from build123d import *

# Parameters (mm, degrees)
F1_DEPTH = 48
F0_W     = 15
F0_H     = 30
F2_DEPTH = 10
F3_R     = 6


with BuildPart() as f1:
    # F0 (on Top) → F1 (new body)
    with BuildSketch(Plane.XY):
        Polygon((21, 30), (21, 10), (-21, 10), (-21, 30), (-31, 30), (-31, 0), (31, 0), (31, 30), align=None)
    extrude(amount=F1_DEPTH)

    # F0 (on Top) → F2 (join)
    with BuildSketch(Plane.XY):
        Polygon((46, 0), (31, 0), (-31, 0), (-46, 0), (-46, -18), (46, -18), align=None)
        with Locations((38.5, 15)):
            Rectangle(F0_W, F0_H)
        with Locations((-38.5, 15)):
            Rectangle(F0_W, F0_H)
    extrude(amount=F2_DEPTH)

    # F3
    f3_edges = [f1.edges().sort_by_distance(p)[0] for p in [
        (46, -18, 5),
        (-46, -18, 5),
    ]]
    fillet(f3_edges, radius=F3_R)


solid = f1.part
Source: CAD feature listing. Evaluate the final solid. Frame: model axes, mm. A direction names the side the tool comes from. Coordinates: 2 decimals unless noted, no trailing zeros. Loops run counter-clockwise (first coordinate to the right, second up) from the corner with the lowest first, then second, coordinate; pieces in that order, holes last. Notation, with made-up numbers: (14.5, 79) - (23.5, 79) arc R9 cw to (23.5, 91) - close; hole circle Ø5 at (38, 25.5). An arc over 180 degrees is marked (long way). One line per item, written item: value. Start each with the question number.
1. Contact query for flat-ended pins moving along their axis: P1, Ø11.5, axis at x = -14.5, z = 33.5, coming from the -Y side; P2, Ø2, axis at x = -30.5, y = 16, coming from the -Z side; P3, Ø9, axis at y = 21, z = 32, coming from the -X side; P4, Ø15, axis at y = 13, z = 36, coming from the +X side. Output: stop coordinate, or through.
2. Ray query, L1, parallel to X at y = 17.5, z = 40.5; L2, parallel to Y at x = -6, z = 33.5. Return the intervals inside material, ascending.
3. Mould query, pull axis X, two halves, no side actions, for faces 1 (the flat face through (-31, 15, 29)), 2 (the flat face through (-21, 20, 24)), 3 (the cylindrical face through (44.289, -16.196, 5.07)). Classes: pulls with the +X half, pulls with the -X half, needs draft (parallel to the pull), parting line crosses it, or undercut.
4. Set-up query: faces 4 (the flat face through (0, 10, 24)), 5 (the flat face through (0, 0, 29)), 6 (the flat face through (31, 15, 29)). Return all of +Z, -Z, +X, -X, +Y, -Y with unobstructed straight access to the full face (end or side cutting, diameter ignored); none if empty.
5. Section D-D (y = 4.5). Return the cut outline in (x, z).
6. Section C-C (x = -28). Return the cut outline in (y, z), and give its area (3 significant figures).
7. Section A-A (y = 13.5). Return the cut outline in (x, z), and give its area (3 significant figures).
8. Section B-B (z = 29.5). Return the cut outline in (x, y), and give its area (3 significant figures).
Verdict:
1. P1: stops at y = 0
1. P2: stops at z = 0
1. P3: stops at x = -31
1. P4: stops at x = 31
2. L1: x = -31 to -21, 21 to 31
2. L2: y = 0 to 10
3. face 1: pulls with the -X half
3. face 2: undercut
3. face 3: pulls with the +X half
4. face 4: +Z, -Z, +Y
4. face 5: +Z, +X, -X, -Y
4. face 6: +Z, +X, +Y, -Y
5. outline: (-46, 0) - (46, 0) - (46, 10) - (31, 10) - (31, 48) - (-31, 48) - (-31, 10) - (-46, 10) - close
6. outline: (-18, 0) - (30, 0) - (30, 48) - (0, 48) - (0, 10) - (-18, 10) - close
6. area: 1,620 mm2
7. outline: (-46, 0) - (-21, 0) - (-21, 48) - (-31, 48) - (-31, 10) - (-46, 10) - close; (21, 0) - (46, 0) - (46, 10) - (31, 10) - (31, 48) - (21, 48) - close
7. area: 1,260 mm2
8. outline: (-31, 0) - (31, 0) - (31, 30) - (21, 30) - (21, 10) - (-21, 10) - (-21, 30) - (-31, 30) - close
8. area: 1,020 mm2
